Design review of the part built by this model. Coordinates are the model's own, in mm. A direction names the side the tool comes from. Round coordinates to 2 decimals unless told otherwise and drop trailing zeros. Loops run counter-clockwise (first coordinate to the right, second up) from the corner with the lowest first, then second, coordinate; pieces in that order, holes last. Notation, with made-up numbers: (56.25, 80) -> (102.25, 80) arc R27 cw to (102.25, 107) -> close; hole circle Ø3 at (15.5, 46). An arc over 180 degrees is marked (long way). Answer as CSV lines item,"result". Start each with the question number.
(1) For P1, Ø12.5, axis at x = -16, y = -14.5, coming from the +Z side; P2, Ø5, axis at x = 9.5, z = 17, coming from the +Y side; P3, Ø5, axis at y = 13, z = 25, coming from the +X side; P4, Ø12, axis at y = 5.5, z = 13, coming from the +X side, all flat-tipped, find the tip position at first contact; note any pin that passes through.
(2) Take a section at A-A, the plane y = 10. Write out the cut boundary in (x, z), and give its area (3 significant figures).
(3) To check wall thickness, follow line 1 (Z direction, x = -11.5, y = -11.5); line 2 (X direction, y = 10, z = 26.7); line 3 (Y direction, x = -19.5, z = 22). State the ranges of each line that lie inside material, in increasing order. Write a range as from..to.
(4) Take a section at B-B, the plane y = -4.5. Write out the cut boundary in (x, z), and give its area (3 significant figures).
(5) Take a section at C-C, the plane z = 1. Write out the cut boundary in (x, y).
(6) Take a section at D-D, the plane x = -14. Write out the cut boundary in (y, z).
(7) Machinability: for faces 4 (the face through (16.775, -24, -1)), 5 (the face through (-10, -2, 24)), 6 (the face through (-12.1, 7.6, 25.161)), 7 (the face through (-29.725, -13, -22)), 8 (the face through (20, -14, -16.339)), which of the approach directions +Z, -Z, +X, -X, +Y, -Y give a long, thin tool a straight path to every point of the face, cutting with its end or side? Answer none if there is none.
(8) Draft analysis for pull direction X (two halves, no side actions). For faces 1 (the face through (-35.225, -24, -11)), 2 (the face through (-10, 0, 1)), 3 (the face through (10.275, -13, -22)), state which applies: +X half, -X half, draft (parallel to the pull), parting line (faces both ways), or undercut.
from build123d import *

# Parameters (mm, degrees)
F0_W      = 60
F0_H      = 44.5
F1_DEPTH  = 2
F2_W      = 40
F2_H      = 2
F2_W_2    = 2
F2_H_2    = 30.5
F2_H_3    = 10
F3_DEPTH  = 23
F4_W      = 40
F4_H      = 2
F5_DEPTH  = 4
F6_W      = 2
F6_H      = 10
F7_DEPTH  = 4
F8_W      = 40
F8_H      = 2
F9_DEPTH  = 4
F10_W     = 2
F10_H     = 30.5
F11_DEPTH = 4
F12_W     = 20
F12_H     = 2
F13_DEPTH = 6
F14_W     = 20
F14_H     = 2
F15_DEPTH = 22
F16_R     = 3
F17_DEPTH = 3


with BuildPart() as f1:
    # F0 (on Front) → F1 (new body)
    with BuildSketch(Plane.XZ):
        with Locations((-9.224907, -1.08871)):
            Rectangle(F0_W, F0_H)
    extrude(amount=F1_DEPTH)

    # F2 (on face) → F3 (join)
    with BuildSketch(Plane.XZ.offset(2)):
        with Locations((-8.724907, 20.16129)):
            Rectangle(F2_W, F2_H)
        with Locations((-9.724907, -22.33871)):
            Rectangle(F2_W, F2_H)
        with Locations((19.775093, -1.08871)):
            Rectangle(F2_W_2, F2_H_2)
        with Locations((-38.224907, 9.16129)):
            Rectangle(F2_W_2, F2_H_3)
        with Locations((-38.224907, -11.33871)):
            Rectangle(F2_W_2, F2_H_3)
    extrude(amount=F3_DEPTH)

    # F4 (on face) → F5 (join)
    with BuildSketch(Plane(origin=(0, 0, -23.33871), x_dir=(1, 0, 0), z_dir=(0, 0, -1))):
        with Locations((-9.724907, 24)):
            Rectangle(F4_W, F4_H)
    extrude(amount=-F5_DEPTH)

    # F6 (on face) → F7 (join)
    with BuildSketch(Plane(origin=(-39.224907, 0, 0), x_dir=(0, -1, 0), z_dir=(-1, 0, 0))):
        with Locations((24, 9.16129)):
            Rectangle(F6_W, F6_H)
        with Locations((24, -11.33871)):
            Rectangle(F6_W, F6_H)
    extrude(amount=-F7_DEPTH)

    # F8 (on face) → F9 (join)
    with BuildSketch(Plane.XY.offset(21.16129)):
        with Locations((-8.724907, -24)):
            Rectangle(F8_W, F8_H)
    extrude(amount=-F9_DEPTH)

    # F10 (on face) → F11 (join)
    with BuildSketch(Plane.YZ.offset(20.775093)):
        with Locations((-24, -1.08871)):
            Rectangle(F10_W, F10_H)
    extrude(amount=-F11_DEPTH)

    # F12 (on face) → F13 (join)
    with BuildSketch(Plane.XY.offset(21.16129)):
        with Locations((-9.724907, -1)):
            Rectangle(F12_W, F12_H)
    extrude(amount=F13_DEPTH)

    # F14 (on face) → F15 (join)
    with BuildSketch(Plane.XZ.offset(2)):
        with Locations((-9.724907, 26.16129)):
            Rectangle(F14_W, F14_H)
    extrude(amount=-F15_DEPTH)

    # F16 (on face) → F17 (cut)
    with BuildSketch(Plane(origin=(0, 0, 25.16129), x_dir=(1, 0, 0), z_dir=(0, 0, -1))):
        with Locations((-9.724907, -10)):
            Circle(F16_R)
    extrude(amount=-F17_DEPTH, mode=Mode.SUBTRACT)


solid = f1.part
The answers:
1,P1,"z = 21.16"
1,P2,"y = 0"
1,P3,"x = 0.28"
1,P4,"x = 20.78"
2,outline,"(-19.72, 25.16) -> (-12.72, 25.16) -> (-12.72, 27.16) -> (-19.72, 27.16) -> close; (-6.72, 25.16) -> (0.28, 25.16) -> (0.28, 27.16) -> (-6.72, 27.16) -> close"
2,area,"28.0 mm²"
3,line 1,"-23.34..-21.34, 19.16..21.16"
3,line 2,"-19.72..-12.72, -6.72..0.28"
3,line 3,"-2..0"
4,outline,"(-39.22, -16.34) -> (-37.22, -16.34) -> (-37.22, -6.34) -> (-39.22, -6.34) -> close; (-39.22, 4.16) -> (-37.22, 4.16) -> (-37.22, 14.16) -> (-39.22, 14.16) -> close; (-29.72, -23.34) -> (10.28, -23.34) -> (10.28, -21.34) -> (-29.72, -21.34) -> close; (-28.72, 19.16) -> (11.28, 19.16) -> (11.28, 21.16) -> (-28.72, 21.16) -> close; (18.78, -16.34) -> (20.78, -16.34) -> (20.78, 14.16) -> (18.78, 14.16) -> close"
4,area,"261 mm²"
5,outline,"(-39.22, -2) -> (18.78, -2) -> (18.78, -23) -> (16.78, -23) -> (16.78, -25) -> (20.78, -25) -> (20.78, 0) -> (-39.22, 0) -> close"
6,outline,"(-25, -23.34) -> (0, -23.34) -> (0, 25.16) -> (20, 25.16) -> (20, 27.16) -> (-2, 27.16) -> (-2, 21.16) -> (-25, 21.16) -> (-25, 17.16) -> (-23, 17.16) -> (-23, 19.16) -> (-2, 19.16) -> (-2, -21.34) -> (-23, -21.34) -> (-23, -19.34) -> (-25, -19.34) -> close"
7,face 4,"+Z, -Z, -Y"
7,face 5,"+Z, +X, -X, -Y"
7,face 6,"-Z, +X, -X, +Y"
7,face 7,"+Z, -Z, -X, -Y"
7,face 8,"-Z, +X, -X, -Y"
8,face 1,"undercut"
8,face 2,"draft"
8,face 3,"+X half"
